Study the drawing (mm; zero at the part's minimum x, y, z) and answer. A direction names the side the tool comes from. Round coordinates to 2 decimals unless told otherwise and drop trailing zeros. Loops run counter-clockwise (first coordinate to the right, second up) from the corner with the lowest first, then second, coordinate; pieces in that order, holes last. Notation, with made-up numbers: (67, 72.5) -> (81, 72.5) arc R18 cw to (81, 102.5) -> close; hole circle Ø3 at (-28.5, 1). An arc over 180 degrees is marked (long way). Use one line per item in the form item = value.
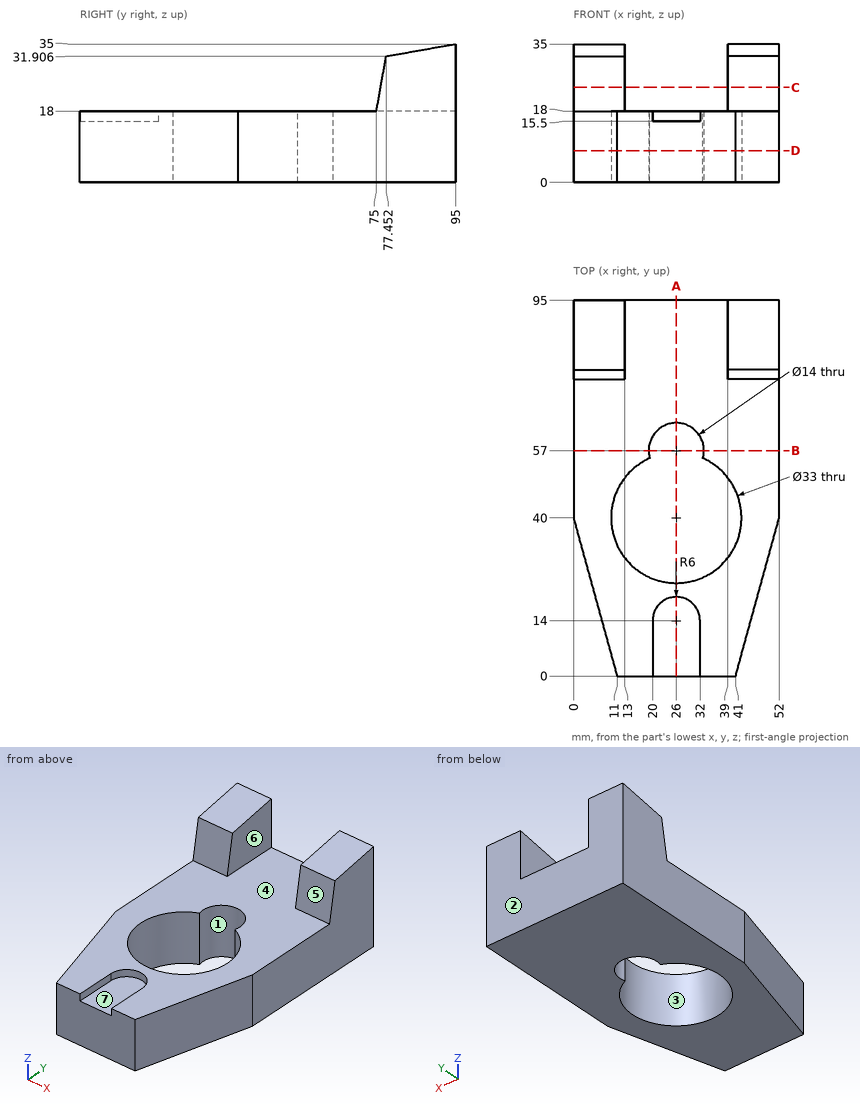
(1) Find section B-B, the plane y = 57. Write down the section's boundary in (x, z).
Completed:
outline = (0, 0) -> (19, 0) -> (19, 18) -> (0, 18) -> close; (33, 0) -> (52, 0) -> (52, 18) -> (33, 18) -> close
(2) Find section A-A, the plane x = 26. Write down the section's boundary in (y, z), then the cut area to 3 significant figures.
Completed:
outline = (0, 0) -> (23.5, 0) -> (23.5, 18) -> (20, 18) -> (20, 15.5) -> (0, 15.5) -> close; (64, 0) -> (95, 0) -> (95, 18) -> (64, 18) -> close
area = 931 mm2
(3) Given P1, Ø13.5, axis at y = 87.5, z = 26, coming from the -X side; P2, Ø6, axis at x = 30, y = 80.5, coming from the +Z side; P3, Ø6, axis at x = 24.5, y = 14, coming from the +Z side; P4, Ø6, axis at x = 10.5, z = 31.5, coming from the -Y side, each flat-ended and moving along its own axis, determine where each tip first touches the part or whether it passes through.
Completed:
P1 = 0
P2 = 18
P3 = 15.5
P4 = 76.85
(4) For the marked faces 5, 6 and 7, determine the directions among +Z, -Z, +X, -X, +Y, -Y from which every point of the face is accessible in a straight line to the end or side of a thin tool.
Completed:
face_5 = +Z, +X, -X, -Y
face_6 = +Z, +Y, -Y
face_7 = +Z, -Y
(5) Find section C-C, the plane z = 24. Write down the section's boundary in (x, y).
Completed:
outline = (0, 76.06) -> (13, 76.06) -> (13, 95) -> (0, 95) -> close; (39, 76.06) -> (52, 76.06) -> (52, 95) -> (39, 95) -> close
(6) For a pull along Y with two mould halves and no side action, classify the marked faces 1, 2, 3 and 4 as +Y half, -Y half, draft (parallel to the pull), parting line (faces both ways), or undercut.
Completed:
face_1 = undercut
face_2 = +Y half
face_3 = undercut
face_4 = draft
(7) Find section D-D, the plane z = 8. Write down the section's boundary in (x, y), then the cut area to 3 significant figures.
Completed:
outline = (0, 40) -> (11, 0) -> (41, 0) -> (52, 40) -> (52, 95) -> (0, 95) -> close; hole (19.27, 55.07) arc R16.5 ccw (long way) to (32.73, 55.07) arc R7 ccw (long way) to start
area = 3,550 mm2
(8) Consider L1, parallel to X at y = 57, z = 13; L2, parallel to X at y = 40, z = 14.75; L3, parallel to Z at x = 16.5, y = 14. Determine where each line is inside the solid, lowest interval first.
Completed:
L1 = 0 to 19, 33 to 52
L2 = 0 to 9.5, 42.5 to 52
L3 = 0 to 18
